Autodesk Fusion 360 part; units mm, degrees
sketch "Sketch1" plane through (0, 0, 0) normal (0, 1, 0) x (1, 0, 0)
  line L0 (60.5, -38) -> (-60.5, -38)
  line L1 (-60.5, -38) -> (-60.5, 38)
  line L2 (-60.5, 38) -> (60.5, 38)
  line L3 (60.5, 38) -> (60.5, -38)
  line L4 (60.5, -38) -> (-60.5, 38) construction
  line L5 (-60.5, -38) -> (60.5, 38) construction
  line L6 (56.5, -34) -> (-56.5, -34) construction
  line L7 (-56.5, -34) -> (-56.5, 34) construction
  line L8 (-56.5, 34) -> (56.5, 34) construction
  line L9 (56.5, 34) -> (56.5, -34) construction
  line L10 (56.5, -34) -> (-56.5, 34) construction
  line L11 (-56.5, -34) -> (56.5, 34) construction
  circle A0 centre (56.5, 34) radius 3
  circle A1 centre (56.5, -34) radius 3
  circle A2 centre (-56.5, -34) radius 3
  circle A3 centre (-56.5, 34) radius 3
  dimension "d1" = 121
  dimension "d2" = 76
  dimension "d3" = 113
  dimension "d4" = 68
  dimension "d5" = 6
  dimension "d6" = 6
  dimension "d7" = 6
  dimension "d8" = 6
extrude "Extrude1" add sketch "Sketch1" along normal blind 10
extrude "Extrude2" add sketch "Sketch1" along normal blind 14.2 contours A0 | A1 | A2 | A3
equation "d11 = 10 mm + 4.2 mm"
Can you work these out from the model? Positions are in its coordinate system, mm. A direction names the side the tool comes from. Coordinates: 2 decimals unless noted, no trailing zeros. Write each loop counter-clockwise with the first axis right and the second up, starting at its lowest first coordinate (ties: lowest second). Pieces come first, ordered by that corner, then holes. Notation, with made-up numbers: (-1.5, 17) -> (45.5, 17) arc R5 cw to (45.5, 22) -> close; hole circle Ø6 at (-7, 82). An arc over 180 degrees is marked (long way). Write each question's results on one line, items separated by ' | '. Start each with the question number.
Q1. Imagine slicing it at A-A (z = 34). Write out the boundary of the cut face in (x, y), then the cut area to 3 significant figures.
Q2. Imagine slicing it at C-C (x = 56.5). Write out the boundary of the cut face in (y, z), then the cut area to 3 significant figures.
Q3. We'd pull the mould along X, two halves only. Please class faces 1 (the face through (-59.5, 12.1, 34.1)), 2 (the face through (1, 5, 38)), 3 (the face through (-60.5, 5, 1)): +X half, -X half, draft (parallel to the pull), parting line (faces both ways), or undercut.
Q4. On a 3-axis mill with a long thin cutter (end or side, diameter ignored), from which of +Z, -Z, +X, -X, +Y, -Y can I reach the whole of each face in a straight line? I mean faces 4 (the face through (53.5, 12.1, 34.1)), 5 (the face through (-57, 14.2, -34)). Say none if no direction works.
Q5. I'm going to push a flat-ended pin straight in: pin 1 (10 mm diameter, centred on x = -47, z = -23, fed in from +Y). Where does the tip first touch, or does it pass through?
Q6. If I drill on probe 1 along Y at (x, z) = (-8.5, -30), over which ranges is the centre line in solid material (lowest first)?
Q7. Imagine slicing it at B-B (y = 12.5). Write out the boundary of the cut face in (x, z), then the cut area to 3 significant figures.
Q8. Imagine slicing it at D-D (x = 33). Write out the boundary of the cut face in (y, z).
Taken from the geometry:
1) outline: (-60.5, 0) -> (60.5, 0) -> (60.5, 10) -> (59.5, 10) -> (59.5, 14.2) -> (53.5, 14.2) -> (53.5, 10) -> (-53.5, 10) -> (-53.5, 14.2) -> (-59.5, 14.2) -> (-59.5, 10) -> (-60.5, 10) -> close | area: 1,260 mm^2
2) outline: (0, -38) -> (10, -38) -> (10, -37) -> (14.2, -37) -> (14.2, -31) -> (10, -31) -> (10, 31) -> (14.2, 31) -> (14.2, 37) -> (10, 37) -> (10, 38) -> (0, 38) -> close | area: 810 mm^2
3) face 1: undercut | face 2: draft | face 3: -X half
4) face 4: +Y | face 5: +Z, -Z, +X, -X, +Y
5) pin 1: stops at y = 10
6) probe 1: y = 0 to 10
7) outline: circle Ø6 at (-56.5, -34); circle Ø6 at (-56.5, 34); circle Ø6 at (56.5, -34); circle Ø6 at (56.5, 34) | area: 113 mm^2
8) outline: (0, -38) -> (10, -38) -> (10, 38) -> (0, 38) -> close
